Can you work these out from the model? Positions are in its coordinate system, mm. Give positions to 0.01 mm unless a question says otherwise; leave off trailing zeros. Loops run counter-clockwise (first coordinate to the right, second up) from the corner with the lowest first, then second, coordinate; pieces in that order, holes last. Notation, with made-up numbers: (-14, -5) - (26, -5) arc R18 cw to (26, 26) - close; hole circle Ø7 at (18, 56.25). An arc over 180 degrees is marked (long way). Answer as a JSON object with one key per item and string values. Group by question number.
Item 1: Suppose I cut it at A-A on x = 227. Write out the boundary of the cut face in (y, z).
Item 2: Please list where these lines run through material, in increasing order: L1, parallel to Y at x = 310.5, z = 11.25 (3 decimals); L2, parallel to Y at x = 273, z = 13; L3, parallel to Z at x = 362, y = 4.75 (3 decimals).
Item 3: Suppose I cut it at B-B on z = 5.5. Write out the boundary of the cut face in (x, y).
Item 4: Will these pins go through, and if not, where does the flat tip stop? pin 1 (3 mm diameter, centred on x = 144, y = -6, fed in from -Z); pin 2 (10 mm diameter, centred on x = 92, z = 2.5, fed in from -Y); pin 3 (5 mm diameter, centred on x = 398.5, z = 10.5, fed in from +Y).
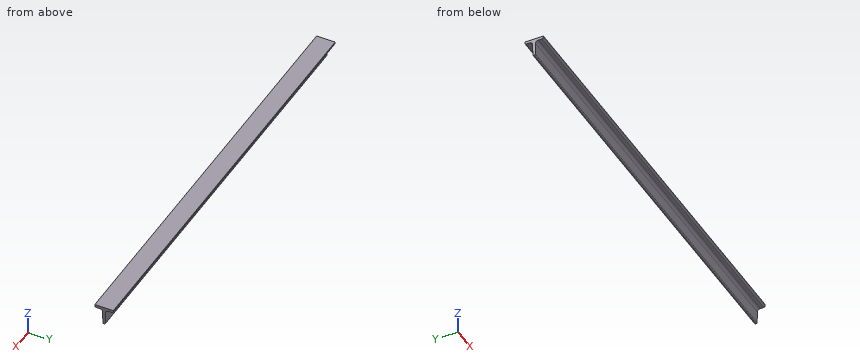
from build123d import *

# Parameters (mm, degrees)
T_SECTION_T_20_X_20_1_DEPTH = 460


with BuildPart() as part:
    # Sketch12 → T section T 20 X 20(1) (new body)
    with BuildSketch(Plane.YZ):
        with BuildLine():
            Line((-10, 20), (10, 20))
            Line((10, 20), (10, 18.570314587))
            ThreePointArc((10, 18.570314587), (9.571214338, 17.520314662), (8.530000209, 17.070614622))
            Line((8.530000209, 17.070614622), (4.520436432, 16.990406743))
            ThreePointArc((4.520436432, 16.990406743), (2.459116507, 16.112327155), (1.581036919, 14.05100723))
            Line((1.581036919, 14.05100723), (1.319562646, 0.97999986))
            ThreePointArc((1.319562646, 0.97999986), (1.019762619, 0.285857108), (0.319762669, 0))
            Line((0.319762669, 0), (-0.319762669, 0))
            ThreePointArc((-0.319762669, 0), (-1.019762619, 0.285857108), (-1.319562646, 0.97999986))
            Line((-1.319562646, 0.97999986), (-1.581036919, 14.05100723))
            ThreePointArc((-1.581036919, 14.05100723), (-2.459116507, 16.112327155), (-4.520436432, 16.990406743))
            Line((-4.520436432, 16.990406743), (-8.530000209, 17.070614622))
            ThreePointArc((-8.530000209, 17.070614622), (-9.571214338, 17.520314662), (-10, 18.570314587))
            Line((-10, 18.570314587), (-10, 20))
        make_face()
    extrude(amount=T_SECTION_T_20_X_20_1_DEPTH)


solid = part.part
Worked out:
{
 "1": {"outline": "(-10, 18.57) arc R1.5 ccw to (-8.53, 17.07) - (-4.52, 16.99) arc R3 cw to (-1.58, 14.05) - (-1.32, 0.98) arc R1 ccw to (-0.32, 0) - (0.32, 0) arc R1 ccw to (1.32, 0.98) - (1.58, 14.05) arc R3 cw to (4.52, 16.99) - (8.53, 17.07) arc R1.5 ccw to (10, 18.57) - (10, 20) - (-10, 20) - close"},
 "2": {"L1": "y = -1.525 to 1.525", "L2": "y = -1.56 to 1.56", "L3": "z = 16.995 to 20"},
 "3": {"outline": "(0, -1.41) - (460, -1.41) - (460, 1.41) - (0, 1.41) - close"},
 "4": {"pin 1": "stops at z = 16.99", "pin 2": "stops at y = -1.45", "pin 3": "stops at y = 1.56"}
}
